Design review of the part built by this model. Coordinates are the model's own, in mm. Round coordinates to 2 decimals unless told otherwise and drop trailing zeros. Write item = value, one per line. Start each with the question number.
```python
from build123d import *

# Parameters (mm, degrees)
SKETCH1_R           = 44.45
BOSS_EXTRUDE1_DEPTH = 2.54
SKETCH2_R           = 1.5875
CUT_EXTRUDE1_DEPTH  = 64.066721811
FILLET1_R           = 1.5875


with BuildPart() as part:
    # Sketch1 → Boss-Extrude1 (new, symmetric)
    with BuildSketch(Plane.XY):
        Circle(SKETCH1_R)
        with BuildLine():
            Line((1.248223297, 1.0414), (-1.248223297, 1.0414))
            ThreePointArc((-1.248223297, 1.0414), (0, -1.6256), (1.248223297, 1.0414))
        make_face(mode=Mode.SUBTRACT)
    extrude(amount=BOSS_EXTRUDE1_DEPTH, both=True)

    # Sketch2 → Cut-Revolve1 (revolve, cut)
    with BuildSketch(Plane(origin=(0, 0, 0), x_dir=(1, 0, 0), z_dir=(0, 1, 0))):
        with Locations((44.45, 0)):
            Circle(SKETCH2_R)
    revolve(axis=Axis((0, 0, 0), (0, 0, -1)), mode=Mode.SUBTRACT)

    # Sketch4 → Cut-Extrude1 (cut, through all)
    with BuildSketch(Plane.XY.offset(2.54)):
        with BuildLine():
            ThreePointArc((-3.785529256, 3.900707066), (-3.194965517, 4.397492775), (-2.54, 4.80563704))
            Line((-2.54, 4.80563704), (-1.5875, 39.337980931))
            ThreePointArc((-1.5875, 39.337980931), (-23.141105383, 31.850999069), (-36.922078624, 13.665906852))
            Line((-36.922078624, 13.665906852), (-3.785529256, 3.900707066))
        make_face()
        with BuildLine():
            Line((1.5875, 39.337980931), (2.54, 4.80563704))
            ThreePointArc((2.54, 4.80563704), (3.194965517, 4.397492775), (3.785529256, 3.900707066))
            Line((3.785529256, 3.900707066), (36.922078624, 13.665906852))
            ThreePointArc((36.922078624, 13.665906852), (23.141105383, 31.850999069), (1.5875, 39.337980931))
        make_face()
        with BuildLine():
            ThreePointArc((39.37, 0), (39.001578061, 5.373435471), (37.903207581, 10.646302413))
            Line((37.903207581, 10.646302413), (5.355335588, -0.930660037))
            ThreePointArc((5.355335588, -0.930660037), (5.1695628, -1.679692775), (4.879585746, -2.394867493))
            Line((4.879585746, -2.394867493), (24.406599525, -30.89198601))
            ThreePointArc((24.406599525, -30.89198601), (35.432222082, -17.162591248), (39.37, 0))
        make_face()
        with BuildLine():
            ThreePointArc((0.769779414, -5.380816575), (0, -5.4356), (-0.769779414, -5.380816575))
            Line((-0.769779414, -5.380816575), (-21.837970568, -32.758204186))
            ThreePointArc((-21.837970568, -32.758204186), (0, -39.37), (21.837970568, -32.758204186))
            Line((21.837970568, -32.758204186), (0.769779414, -5.380816575))
        make_face()
        with BuildLine():
            ThreePointArc((-4.879585746, -2.394867493), (-5.1695628, -1.679692775), (-5.355335588, -0.930660037))
            Line((-5.355335588, -0.930660037), (-37.903207581, 10.646302413))
            ThreePointArc((-37.903207581, 10.646302413), (-37.443095047, -12.165999069), (-24.406599525, -30.89198601))
            Line((-24.406599525, -30.89198601), (-4.879585746, -2.394867493))
        make_face()
    extrude(amount=-CUT_EXTRUDE1_DEPTH, mode=Mode.SUBTRACT)

    # Fillet1
    fillet1_edges = [part.edges().sort_by_distance(p)[0] for p in [
        (24.406599525, -30.89198601, 0),
        (4.879585746, -2.394867493, 0),
        (5.355335588, -0.930660037, 0),
        (37.903207581, 10.646302413, 0),
        (36.922078624, 13.665906852, 0),
        (3.785529256, 3.900707066, 0),
        (2.54, 4.80563704, 0),
        (1.5875, 39.337980931, 0),
        (-37.903207581, 10.646302413, 0),
        (-5.355335588, -0.930660037, 0),
        (-4.879585746, -2.394867493, 0),
        (-24.406599525, -30.89198601, 0),
        (-21.837970568, -32.758204186, 0),
        (-0.769779414, -5.380816575, 0),
        (0.769779414, -5.380816575, 0),
        (21.837970568, -32.758204186, 0),
        (-1.5875, 39.337980931, 0),
        (-2.54, 4.80563704, 0),
        (-3.785529256, 3.900707066, 0),
        (-36.922078624, 13.665906852, 0),
    ]]
    fillet(fillet1_edges, radius=FILLET1_R)


solid = part.part
```
(1) Consider section A-A, the plane x = 9.5. State how many separate pieces and enclosed holes the cut face has, then the cut area to 3 significant figures.
(2) Draft analysis for pull direction Y (two halves, no side actions). For faces 1 (the face through (0, 4, 2.54)), 2 (the face through (11.17, -18.895, 0.036)), 3 (the face through (42.397, 13.352, -2.057)), state which applies: pulls with the +Y half, pulls with the -Y half, needs draft (parallel to the pull), parting line crosses it, or undercut.
(3) Insertion check: pin 1 (2 mm diameter, centred on x = 0, z = 0, fed in from -Y); pin 2 (3 mm diameter, centred on x = 19, z = 0.5, fed in from +Y). Each pin has a flat end and moves straight along its axis. Give the tip position at first contact, or say it passes through.
(4) For line 1 along Y through (x, z) = (-12, -2.15); line 2 along X through (y, z) = (-16, 1.65); line 3 along Y through (x, z) = (-10, -1), list the stretches that pass through material, from the lowest coordinate up. Write a range as [from, to].
Completed:
q1.separate_pieces = 4
q1.enclosed_holes = 0
q1.area = 109 mm2
q2.face_1 = needs draft
q2.face_2 = undercut
q2.face_3 = parting line crosses it
q3.pin_1 = -43.22
q3.pin_2 = 40.66
q4.line_1 = [-42.8, -37.5], [-19.97, -12.79], [1.43, 6.32], [37.5, 42.8]
q4.line_2 = [-41.47, -35.97], [-14.2, -8.94], [8.94, 14.2], [35.97, 41.47]
q4.line_3 = [-42.04, -38.08], [-17.38, -9.87], [0.72, 5.73], [38.08, 42.04]
